Source: CAD feature listing. Evaluate the final solid. Frame: model axes, mm. A direction names the side the tool comes from. Give positions to 0.01 mm unless a question says otherwise; leave off trailing zeros. Write each loop counter-clockwise with the first axis right and the second up, starting at its lowest first coordinate (ties: lowest second). Pieces come first, ordered by that corner, then holes. Notation, with made-up numbers: (78.5, 10.25) - (105.5, 10.25) arc R33 cw to (105.5, 49.25) - close; hole circle Ø9 at (8.5, 82.5). An arc over 180 degrees is marked (long way). Answer as a JSON object with one key per item and string values. Group by question number.
from build123d import *

# Parameters (mm, degrees)
CROQUIS1_R                 = 18
CROQUIS1_R_2               = 15.5
SALIENTE_EXTRUIR1_DEPTH    = 15
CROQUIS2_R                 = 20
CROQUIS2_R_2               = 15.5
SALIENTE_EXTRUIR2_DEPTH    = 3.5
CROQUIS4_R                 = 16.5
CROQUIS4_R_2               = 13.5
SALIENTE_EXTRUIR3_DEPTH    = 4
CROQUIS5_R                 = 16.5
SALIENTE_EXTRUIR4_DEPTH    = 3
SALIENTE_EXTRUIR5_DEPTH    = 31
CROQUIS7_R                 = 15
CROQUIS8_R                 = 19
CROQUIS9_R                 = 13
CROQUIS10_R                = 17
CORTAR_EXTRUIR1_DEPTH      = 41
CORTAR_EXTRUIR1_DEPTH_BACK = 13
CROQUIS12_R                = 15
SALIENTE_EXTRUIR6_DEPTH    = 2
CROQUIS14_R                = 11
SALIENTE_EXTRUIR7_DEPTH    = 22
SALIENTE_EXTRUIR7_TAPER    = 2
CROQUIS17_R                = 9
CROQUIS15_R                = 8.231743071
CROQUIS18_R                = 9
CORTAR_EXTRUIR2_DEPTH      = 57
CROQUIS19_R                = 10.231743071
SALIENTE_EXTRUIR8_DEPTH    = 2
CROQUIS20_R                = 23.75
CROQUIS20_R_2              = 17
SALIENTE_EXTRUIR9_DEPTH    = 3.5


with BuildPart() as part:
    # Croquis1 → Saliente-Extruir1 (new body)
    with BuildSketch(Plane(origin=(0, 0, 0), x_dir=(0, 0, -1), z_dir=(1, 0, 0))):
        Circle(CROQUIS1_R)
        Circle(CROQUIS1_R_2, mode=Mode.SUBTRACT)
    extrude(amount=SALIENTE_EXTRUIR1_DEPTH)

    # Croquis2 → Saliente-Extruir2 (add)
    with BuildSketch(Plane(origin=(15, 0, 0), x_dir=(0, 0, -1), z_dir=(1, 0, 0))):
        Circle(CROQUIS2_R)
        Circle(CROQUIS2_R_2, mode=Mode.SUBTRACT)
    extrude(amount=SALIENTE_EXTRUIR2_DEPTH)

    # Croquis4 → Saliente-Extruir3 (add)
    with BuildSketch(Plane(origin=(18.5, 0, 0), x_dir=(0, 0, -1), z_dir=(1, 0, 0))):
        Circle(CROQUIS4_R)
        Circle(CROQUIS4_R_2, mode=Mode.SUBTRACT)
    extrude(amount=SALIENTE_EXTRUIR3_DEPTH)

    # Croquis5 → Saliente-Extruir4 (add)
    with BuildSketch(Plane(origin=(22.5, 0, 0), x_dir=(0, 0, -1), z_dir=(1, 0, 0))):
        Circle(CROQUIS5_R)
    extrude(amount=-SALIENTE_EXTRUIR4_DEPTH)

    # Croquis6 → Saliente-Extruir5 (add)
    with BuildSketch(Plane(origin=(22.5, 0, 0), x_dir=(0, 0, -1), z_dir=(1, 0, 0))):
        with BuildLine():
            Line((-7.5, 7.5), (-7.5, -7.5))
            ThreePointArc((-7.5, -7.5), (0, -10.5), (7.5, -7.5))
            Line((7.5, -7.5), (7.5, 7.5))
            ThreePointArc((7.5, 7.5), (0, 10.5), (-7.5, 7.5))
        make_face()
        with BuildLine():
            Line((-5.5, 6.590315858), (-5.5, -6.590315858))
            ThreePointArc((-5.5, -6.590315858), (0, -8.5), (5.5, -6.590315858))
            Line((5.5, -6.590315858), (5.5, 6.590315858))
            ThreePointArc((5.5, 6.590315858), (0, 8.5), (-5.5, 6.590315858))
        make_face(mode=Mode.SUBTRACT)
    extrude(amount=SALIENTE_EXTRUIR5_DEPTH)

    # Croquis7 → Recubrir1 section 0
    with BuildSketch(Plane.XY.offset(7.5)):
        with Locations((64.212142643, 0)):
            Circle(CROQUIS7_R)
    # Croquis8 → Recubrir1 section 1
    with BuildSketch(Plane.XY.offset(-14.5)):
        with Locations((64.212142643, 0)):
            Circle(CROQUIS8_R)
    loft()

    # Croquis9 → Cortar-Recubrir1 section 0
    with BuildSketch(Plane.XY.offset(7.5)):
        with Locations((64.212142643, 0)):
            Circle(CROQUIS9_R)
    # Croquis10 → Cortar-Recubrir1 section 1
    with BuildSketch(Plane(origin=(0, 0, -14.5), x_dir=(-1, 0, 0), z_dir=(0, 0, -1))):
        with Locations((-64.212142643, 0)):
            Circle(CROQUIS10_R)
    loft(mode=Mode.SUBTRACT)

    # Croquis11 → Cortar-Extruir1 (cut, two sides)
    with BuildSketch(Plane(origin=(22.5, 0, 0), x_dir=(0, 0, -1), z_dir=(1, 0, 0))) as cortar_extruir1_sk:
        with BuildLine():
            Line((-5.5, 6.590315858), (-5.5, -6.590315858))
            ThreePointArc((-5.5, -6.590315858), (0, -8.5), (5.5, -6.590315858))
            Line((5.5, -6.590315858), (5.5, 6.590315858))
            ThreePointArc((5.5, 6.590315858), (0, 8.5), (-5.5, 6.590315858))
        make_face()
    extrude(amount=CORTAR_EXTRUIR1_DEPTH, mode=Mode.SUBTRACT)
    extrude(cortar_extruir1_sk.sketch, amount=-CORTAR_EXTRUIR1_DEPTH_BACK, mode=Mode.SUBTRACT)

    # Croquis12 → Saliente-Extruir6 (add)
    with BuildSketch(Plane.XY.offset(7.5)):
        with Locations((64.212142643, 0)):
            Circle(CROQUIS12_R)
    extrude(amount=-SALIENTE_EXTRUIR6_DEPTH)

    # Croquis14 → Saliente-Extruir7 (add)
    with BuildSketch(Plane(origin=(0, 0, 5.5), x_dir=(-1, 0, 0), z_dir=(0, 0, -1))):
        with Locations((-64.212142643, 0)):
            Circle(CROQUIS14_R)
    extrude(amount=SALIENTE_EXTRUIR7_DEPTH, taper=SALIENTE_EXTRUIR7_TAPER)

    # Croquis17 → Cortar-Recubrir2 section 0
    with BuildSketch(Plane(origin=(0, 0, 5.5), x_dir=(-1, 0, 0), z_dir=(0, 0, -1))):
        with Locations((-64.212142643, 0)):
            Circle(CROQUIS17_R)
    # Croquis15 → Cortar-Recubrir2 section 1
    with BuildSketch(Plane(origin=(0, 0, -16.5), x_dir=(-1, 0, 0), z_dir=(0, 0, -1))):
        with Locations((-64.212142643, 0)):
            Circle(CROQUIS15_R)
    loft(mode=Mode.SUBTRACT)

    # Croquis18 → Cortar-Extruir2 (cut)
    with BuildSketch(Plane(origin=(0, 0, 5.5), x_dir=(-1, 0, 0), z_dir=(0, 0, -1))):
        with Locations((-64.212142643, 0)):
            Circle(CROQUIS18_R)
    extrude(amount=-CORTAR_EXTRUIR2_DEPTH, mode=Mode.SUBTRACT)

    # Croquis19 → Saliente-Extruir8 (add)
    with BuildSketch(Plane(origin=(0, 0, -16.5), x_dir=(-1, 0, 0), z_dir=(0, 0, -1))):
        with Locations((-64.212142643, 0)):
            Circle(CROQUIS19_R)
    extrude(amount=-SALIENTE_EXTRUIR8_DEPTH)

    # Croquis20 → Saliente-Extruir9 (add)
    with BuildSketch(Plane(origin=(0, 0, -14.5), x_dir=(-1, 0, 0), z_dir=(0, 0, -1))):
        with Locations((-64.212142643, 0)):
            Circle(CROQUIS20_R)
        with Locations((-64.212142643, 0)):
            Circle(CROQUIS20_R_2, mode=Mode.SUBTRACT)
    extrude(amount=SALIENTE_EXTRUIR9_DEPTH)


solid = part.part
Q1. Section B-B on z = -10. Return the cut outline in (x, y), then the cut area to 3 significant figures.
Q2. Draft query along X for faces 5 (the flat face through (50, 0, 7.5)), 6 (the conical face through (80.03, 4.98, -1.21)), 7 (the flat face through (15, 3, 18)). Return one class per face: released by +X, released by -X, zero draft, split by the parting line, or undercut.
Q3. First-contact query: pin 1 Ø14.5 at (x, y) = (35.5, -1.5) entering from +Z; pin 2 Ø8 at (x, y) = (32.5, -17.5) entering from -Z; pin 3 Ø12 at (y, z) = (-6.5, 15.5) entering from +X; pin 4 Ø13.5 at (y, z) = (6.5, -1) entering from -X. Flat tips, straight axial feed; report the tip coordinate or a pass-through.
Q4. Section A-A on z = 1.5. State how many separate pieces and enclosed holes the cut face has, then the cut area to 3 significant figures.
Q5. Section D-D on z = 14.5. Return the cut outline in (x, y), then the cut area to 3 significant figures.
Q6. Ray query, probe 1 along Y at (x, z) = (19, 0); probe 2 along Y at (x, z) = (66, -9.5); probe 3 along Y at (x, z) = (69, -2). Return the intervals inside material, ascending. Write a range as [from, to].
Q7. Section C-C on x = 26. Return the cut outline in (y, z) (3 decimals), then the cut area to 3 significant figures.
Q8. Reachability of faces 1 (the cylindrical face through (18.99, -13.18, 2.93)), 2 (the cylindrical face through (37.1, -10.5, 0.1)), 3 (the cylindrical face through (70.85, 6.08, 6.49)), 4 (the cylindrical face through (37.1, 10.5, -0.1)) from +Z, -Z, +X, -X, +Y, -Y: full face, straight path, thin tool, end or side. Return the list, or none.
Taken from the geometry:
{
 "1": {"outline": "(0, -14.97) - (15, -14.97) - (15, -17.32) - (18.5, -17.32) - (18.5, -13.12) - (22.5, -13.12) - (22.5, 13.12) - (18.5, 13.12) - (18.5, 17.32) - (15, 17.32) - (15, 14.97) - (0, 14.97) - (0, 11.84) - (18.5, 11.84) - (18.5, 9.07) - (19.5, 9.07) - (19.5, -9.07) - (18.5, -9.07) - (18.5, -11.84) - (0, -11.84) - close; circle Ø36.36 at (64.21, 0); circle Ø20.92 at (64.21, 0); hole circle Ø32.36 at (64.21, 0); hole circle Ø16.92 at (64.21, 0)", "area": "554 mm²"},
 "2": {"face 5": "zero draft", "face 6": "undercut", "face 7": "released by -X"},
 "3": {"pin 1": "stops at z = 7.5", "pin 2": "passes through", "pin 3": "stops at x = 22.5", "pin 4": "stops at x = 19.5"},
 "4": {"separate pieces": "2", "enclosed holes": "1", "area": "555 mm²"},
 "5": {"outline": "(0, -10.67) - (15, -10.67) - (15, -13.77) - (18.5, -13.77) - (18.5, -7.87) - (22.5, -7.87) - (22.5, 7.87) - (18.5, 7.87) - (18.5, 13.77) - (15, 13.77) - (15, 10.67) - (0, 10.67) - (0, 5.48) - (18.5, 5.48) - (18.5, -5.48) - (0, -5.48) - close", "area": "277 mm²"},
 "6": {"probe 1": "y = [-16.5, -13.5], [13.5, 16.5]", "probe 2": "y = [-18, -15.99], [-10.32, -8.29], [8.29, 10.32], [15.99, 18]", "probe 3": "y = [-16.03, -13.93], [-9.61, -7.31], [7.31, 9.61], [13.93, 16.03]"},
 "7": {"outline": "(-7.5, -7.5) - (7.5, -7.5) arc R10.875 ccw to (7.5, 7.5) - (-7.5, 7.5) arc R10.875 ccw to start; hole (-6.59, -5.5) - (6.59, -5.5) arc R8.875 ccw to (6.59, 5.5) - (-6.59, 5.5) arc R8.875 ccw to start", "area": "113 mm²"},
 "8": {"face 1": "-X", "face 2": "-Y", "face 3": "+Z", "face 4": "+Y"}
}
